Verification items for the finished model (mm, model axes). A direction names the side the tool comes from. Round coordinates to 2 decimals unless told otherwise and drop trailing zeros. Loops run counter-clockwise (first coordinate to the right, second up) from the corner with the lowest first, then second, coordinate; pieces in that order, holes last. Notation, with made-up numbers: M 61.5,29.25 L 115.5,29.25 A36 ccw 115.5,67.25 Z; hole C -18.5,82.5 d9. An arc over 180 degrees is marked long. One line per item, written item: value.
Autodesk Inventor part; units mm, degrees
ref_plane "YZ Plane" through (0, 0, 0) normal (1, 0, 0) x (0, 1, 0)
ref_plane "XZ Plane" through (0, 0, 0) normal (0, 1, 0) x (-1, 0, 0)
ref_plane "XY Plane" through (0, 0, 0) normal (0, 0, 1) x (1, 0, 0)
sketch "Sketch1" plane through (0, 0, 0) normal (0, 1, 0) x (-1, 0, 0)
  line L0 (0, 0) -> (0, -60)
  line L1 (0, -60) -> (15, -60)
  line L2 (15, -60) -> (15, 0)
  line L3 (15, 0) -> (0, 0)
  line L4 (7.5, -60) -> (12.5, -60)
  line L5 (12.5, -60) -> (12.5, 0)
  line L6 (7.5, -60) -> (2.5, -60)
  line L7 (2.5, -60) -> (2.5, 0)
  line L8 (12.5, 0) -> (12.5, -2.5)
  line L9 (12.5, -2.5) -> (2.5, -2.5)
  line L10 (12.5, -60) -> (12.5, -57.5)
  line L11 (12.5, -57.5) -> (2.5, -57.5)
  line L12 (15, -60) -> (15, -61)
  line L13 (15, -61) -> (0, -61)
  line L14 (0, -61) -> (0, -60)
  line L15 (12.5, -57.5) -> (12.5, -58.5)
  line L16 (12.5, -58.5) -> (2.5, -58.5)
  dimension "d0" = 60
  dimension "d1" = 15
  dimension "d2" = 5
  dimension "d3" = 5
  dimension "d4" = 2.5
  dimension "d5" = 2.5
  dimension "d12" = 1
  dimension "d13" = 1
extrude "Extrusion1" add sketch "Sketch1" along normal blind 10 contours L3 L7 L1 L0 | L1 L12 L13 L14 | L3 L5 L9 L7 | L7 L16 L5 L1 | L3 L2 L1 L5
sketch "Sketch2" plane through (0, 0, 0) normal (1, 0, 0) x (0, 0, -1)
  line L0 (61, 10) -> (0, 10)
  line L1 (57.5, 0) -> (57.5, 10)
  line L2 (60, 10) -> (57.5, 10)
  line L3 (57.5, 10) -> (57.5, 0)
  line L4 (57.5, 0) -> (47.5, 0)
  line L5 (2.5, 0) -> (58.5, 0)
  line L6 (47.5, 0) -> (47.5, 10)
  line L7 (2.5, 10) -> (58.5, 10)
  line L8 (47.5, 10) -> (57.5, 10)
  line L9 (47.5, 0) -> (57.5, 10)
  line L10 (47.5, 10) -> (57.5, 0)
  circle A0 centre (52.5, 5) radius 1.1
  line L11 (61, 10) -> (60, 10)
  line L12 (60, 10) -> (57.5, 10)
  line L13 (52.5, 5) -> (0, 5)
  line L14 (0, 0) -> (0, 10)
  line L15 (0, 5) -> (2.5, 5)
  line L16 (2.5, 0) -> (2.5, 10)
  line L17 (2.5, 5) -> (22.5, 5)
  circle A1 centre (22.5, 5) radius 1.1
  dimension "d8" = 10
  dimension "d14" = 20
  dimension "d15" = 2.2
extrude "Extrusion2" cut sketch "Sketch2" against normal through all contours A0 L10 L9 | L9 L10 A0 | L10 L13 A0 | A0 L9 L10 | L9 A0 L13 | A1 L13 | L13 A1
properties part number "top"
(1) Sectioned sample at D-D on y = 5. Enter the section's corners in (x, z), and give its area (3 significant figures).
Completed:
outline: M -15,-61 L 0,-61 L 0,-53.6 L -2.5,-53.6 L -2.5,-58.5 L -12.5,-58.5 L -12.5,-53.6 L -15,-53.6 Z; M -15,-51.4 L -12.5,-51.4 L -12.5,-23.6 L -15,-23.6 Z; M -15,-21.4 L -12.5,-21.4 L -12.5,-2.5 L -2.5,-2.5 L -2.5,-21.4 L 0,-21.4 L 0,0 L -15,0 Z; M -2.5,-51.4 L 0,-51.4 L 0,-23.6 L -2.5,-23.6 Z
area: 333 mm^2
(2) Mould release check, pull along Y, two halves, no side actions. Record for faces 3 (the face through (-13.7, 5, -21.4)), 4 (the face through (-2.5, 5, -31)), 5 (the face through (-2, 10, -30)): +Y half, -Y half, draft (parallel to the pull), parting line (faces both ways), or undercut.
Completed:
face 3: undercut
face 4: draft
face 5: +Y half
(3) Tool access check on faces 1 (the face through (-2, 0, -30)), 2 (the face through (-12.5, 5, -31)). Record the directions out of +Z, -Z, +X, -X, +Y, -Y that give a thin tool (end or side, any length) a straight path to the whole face; none if there is none.
Completed:
face 1: +Z, -Z, +X, -X, -Y
face 2: +Y, -Y
(4) Thickness scan on L1, parallel to Z at x = -0.7, y = 5; L2, parallel to Z at x = -8.5, y = 4.75; L3, parallel to Y at x = -13.35, z = -52.5. Record the ranges inside material, lowest first. Write a range as from..to.
Completed:
L1: z = -61..-53.6, -51.4..-23.6, -21.4..0
L2: z = -61..-58.5, -2.5..0
L3: y = 0..3.9, 6.1..10
(5) Sectioned sample at A-A on z = -33.5. Enter the section's corners in (x, y).
Completed:
outline: M -15,0 L -12.5,0 L -12.5,10 L -15,10 Z; M -2.5,0 L 0,0 L 0,10 L -2.5,10 Z
(6) Sectioned sample at B-B on y = 8.75. Enter the section's corners in (x, z).
Completed:
outline: M -15,-61 L 0,-61 L 0,0 L -15,0 Z; hole M -12.5,-58.5 L -2.5,-58.5 L -2.5,-2.5 L -12.5,-2.5 Z
(7) Sectioned sample at C-C on x = -6.5. Enter the section's corners in (y, z).
Completed:
outline: M 0,-61 L 10,-61 L 10,-58.5 L 0,-58.5 Z; M 0,-2.5 L 10,-2.5 L 10,0 L 0,0 Z
